Autodesk Inventor part; units mm, degrees
ref_plane "Work Plane3" through (0, 0, 1.4478) normal (0, 0, -1) x (-1, 0, 0)
ref_plane "YZ Plane" through (0, 0, 0) normal (1, 0, 0) x (0, 1, 0)
ref_plane "XZ Plane" through (0, 0, 0) normal (0, 1, 0) x (-1, 0, 0)
sketch "Sketch1" plane through (0, 0, 0) normal (0, 0, 1) x (1, 0, 0)
  arc A0 (-1.508, 2.794) -> (-1.508, -2.794) centre (0, 0) ccw
  line L0 (-3.175, 0) -> (0, 0) construction
  line L1 (0, 0) -> (3.175, 0) construction
  line L2 (-1.508, 2.794) -> (1.508, 2.794)
  line L3 (-1.508, -2.794) -> (1.508, -2.794)
  arc A1 (1.508, 2.794) -> (-1.508, 2.794) centre (0, 0) ccw construction
  arc A2 (1.508, -2.794) -> (1.508, 2.794) centre (0, 0) ccw
  arc A3 (-1.508, -2.794) -> (1.508, -2.794) centre (0, 0) ccw construction
  circle A4 centre (0, 0) radius 3.429 construction
  circle A5 centre (0, 0) radius 4.064
  circle A6 centre (0, 0) radius 11.1125
  dimension "d1" = 2.794
  dimension "d2" = 3.175
  dimension "d3" = 6.858
  dimension "d5" = 0.635
  dimension "d6" = 22.225
extrude "Extrusion1" add sketch "Sketch1" along normal blind 3.048 contours A5 | A6
sketch "Sketch2" plane through (0, 0, 3.048) normal (0, 0, 1) x (1, 0, 0)
  circle A0 centre (0, 0) radius 11.1125
  arc A1 (-1.508, 2.794) -> (-1.508, -2.794) centre (0, 0) ccw
extrude "Extrusion2" add sketch "Sketch2" along normal blind 3.175
hole "Hole1" at (0, 0, 3.048) direction (0, 0, 1) diameter 3.302 depth 25.4 tip angle 118
sketch "Sketch3" plane through (0, 0, 6.223) normal (0, 0, 1) x (1, 0, 0)
  circle A0 centre (0, 0) radius 11.1125
  circle A1 centre (0, 0) radius 3.429
  circle A2 centre (0, 0) radius 4.064
  dimension "d18" = 6.858
  dimension "d19" = 0.635
extrude "Extrusion3" add sketch "Sketch3" along normal blind 7.2961 contours A0
chamfer "Chamfer1" distance 6.35 distance2 12.3571 1 edges at (-11.1125, 0, 0) measured on face at (0.4465, -5.5398, 0)
sketch "Sketch6" plane through (0, 0, 13.5191) normal (0, 0, 1) x (1, 0, 0)
  circle A0 centre (0, 0) radius 11.1125
  circle A1 centre (0, 0) radius 6.35
  circle A2 centre (0, 0) radius 8.7312
  dimension "d38" = 12.7
  dimension "d52" = 2.3813
  dimension "d53" = 2.3813
extrude "Extrusion5" add sketch "Sketch6" along normal blind 4.9784 contours A2
sketch "Sketch7" plane through (0, 0, 0) normal (1, 0, 0) x (0, 1, 0)
  line L0 (-6.35, 18.4975) -> (6.35, 18.4975)
  line L1 (6.35, 13.5191) -> (-6.35, 13.5191)
  line L2 (0, 0) -> (0, 13.5191) construction
  line L3 (0, 13.5191) -> (0, 18.4975) construction
  point P0 (0, 16.0084)
hole "Hole3" at (0, 0, 16.0084) direction (-1, 0, 0) diameter 2.159 end through all
sketch "Sketch8" plane through (0, 0, 13.5191) normal (0, 0, 1) x (1, 0, 0)
  circle A0 centre (0, 0) radius 11.1125
  circle A1 centre (0, 0) radius 8.7312
  line L0 (-10.3187, 4.1244) -> (-10.3188, -4.1244)
  line L1 (-11.1125, 0) -> (0, 0)
  dimension "d49" = 0.7937
extrude "Extrusion6" cut sketch "Sketch8" against normal through all contours L0 L1 A0 | A0 L1 L0
mirror "Mirror2" about plane through (0, 0, 0) normal (1, 0, 0) of "Hole3", "Extrusion6"
ref_plane "Work Plane3" through (0, 0, 1.4478) normal (0, 0, -1) x (-1, 0, 0)
sketch "Sketch12" plane through (0, 0, 1.4478) normal (0, 0, -1) x (-1, 0, 0)
  circle A0 centre (0, 0) radius 6.35
  circle A1 centre (0, 0) radius 5.0165
  dimension "d60" = 12.7
  dimension "d61" = 10.033
extrude "Extrusion9" add sketch "Sketch12" against normal blind 2.54
sketch "Sketch13" plane through (0, 0, 0) normal (0, 0, -1) x (-1, 0, 0)
  circle A0 centre (0, 0) radius 4.7625
  circle A1 centre (0, 0) radius 5.5065
  circle A2 centre (0, 0) radius 5.1345
  dimension "d64" = 0.372
  dimension "d65" = 0.372
extrude "Extrusion10" cut sketch "Sketch13" against normal up to surface (1.4478 mm away) contours A1
extrude "Extrusion11" add sketch "Sketch13" against normal up to surface (1.4478 mm away) contours A2
equation "\"d52\" = d53"
equation "\"d64\" = d65"
properties part number "Pneumatic Connector -Actuator Side"
Source: CAD feature listing. Evaluate the final solid. Frame: model axes, mm. A direction names the side the tool comes from. Give positions to 0.01 mm unless a question says otherwise; leave off trailing zeros. Write each loop counter-clockwise with the first axis right and the second up, starting at its lowest first coordinate (ties: lowest second). Pieces come first, ordered by that corner, then holes. Notation, with made-up numbers: (77.25, 30.25) - (134.25, 30.25) arc R15 ccw to (134.25, 45.25) - close; hole circle Ø2 at (63.5, -19.75). An arc over 180 degrees is marked (long way). Write item = value, one per line. Start each with the question number.
Q1. Reachability of faces 5 (the flat face through (2, 0, 6.223)), 6 (the flat face through (0, -3, 0)), 7 (the cylindrical face through (1.113, -5.012, 0.714)) from +Z, -Z, +X, -X, +Y, -Y: full face, straight path, thin tool, end or side. Return the list, or none.
Q2. Cut plane C-C, the plane y = 0. Give the number of separate pieces and of enclosed holes in the cut face, then the cut area to 3 significant figures.
Q3. Draft query along Z for faces 1 (the flat face through (-7, 6, 13.519)), 2 (the cylindrical face through (-0.19, 11.11, 12.93)), 3 (the conical face through (6.14, -2.55, 3.67)), 4 (the cylindrical face through (7.51, -0.41, 15.01)). Return one class per face: +Z half, -Z half, draft (parallel to the pull), parting line (faces both ways), or undercut.
Q4. Material intervals for probe 1 along Y at (x, z) = (-0.25, 2); probe 2 along Z at (x, y) = (-5.25, 2.5); probe 3 along Z at (x, y) = (8.25, 0), sorted ascending.
Q5. Pin query (flat end, axial travel): pin 1 Ø6.5 at (x, y) = (-2, 0.5) entering from +Z; pin 2 Ø2.5 at (x, z) = (0, 1) entering from +Y; pin 3 Ø2 at (x, z) = (5.5, 2) entering from +Y; pin 4 Ø1.9 at (y, z) = (0, 16.01) entering from -X. Return the tip coordinate at first contact, or that it passes through.
Q6. Cut plane D-D, the plane z = 9. Return loops of the section in (x, y), then the cut area to 3 significant figures.
Computed values:
q1.face_5 = +Z
q1.face_6 = -Z, +X, -X, +Y, -Y
q1.face_7 = -Z
q2.separate_pieces = 4
q2.enclosed_holes = 0
q2.area = 145 mm²
q3.face_1 = +Z half
q3.face_2 = draft
q3.face_3 = -Z half
q3.face_4 = undercut
q4.probe_1 = -6.35 to -2.79, 2.79 to 6.35
q4.probe_2 = 1.45 to 13.52
q4.probe_3 = 6.79 to 14.93, 17.09 to 18.5
q5.pin_1 = 13.52
q5.pin_2 = 6.35
q5.pin_3 = 4.48
q5.pin_4 = through
q6.outline = circle Ø18.77 at (0, 0); hole circle Ø8.13 at (0, 0)
q6.area = 225 mm²
